Source: CAD feature listing. Evaluate the final solid. Frame: model axes, mm. Face numbers are marked on the shaded views. Give positions to 0.01 mm unless a question says otherwise; leave off trailing zeros. Loops run counter-clockwise (first coordinate to the right, second up) from the corner with the lowest first, then second, coordinate; pieces in that order, holes last. Notation, with made-up numbers: (-32.5, 27.25) -> (9.5, 27.25) arc R24 cw to (9.5, 40.25) -> close; hole circle Ø3 at (49, 20.25). An arc over 180 degrees is marked (long way). Return JSON: item names as keys, results as strings. Group by question number.
(1) Pin query (flat end, axial travel): pin 1 (2 mm diameter, centred on x = -2, z = -3, fed in from -Y); pin 2 (8 mm diameter, centred on x = -12, z = 10, fed in from +Y); pin 3 (1.5 mm diameter, centred on x = 9.5, z = 0.5, fed in from +Y); pin 4 (1.5 mm diameter, centred on y = -4, z = -7, fed in from -X). Return the tip coordinate at first contact, or that it passes through.
(2) Ray query, line 1 (X direction, y = -21, z = -13.25); line 2 (Y direction, x = -4, z = 13.5); line 3 (Z direction, x = -0.5, y = -0.75). Return the intervals inside material, ascending. Write a range as from..to.
(3) Cut plane A-A on y = -26. Return loops of the section in (x, z).
(4) Cut plane B-B on x = 11.5. Return loops of the section in (y, z).
(5) Draft query along X for the marked faces 1, 2 and 3. Return one class per face: released by +X, released by -X, zero draft, split by the parting line, or undercut.
```python
from build123d import *

# Parameters (mm, degrees)
F0_W      = 30
F0_H      = 30
F1_DEPTH  = 30
F2_W      = 25
F2_H      = 25
F2_W_2    = 17
F2_H_2    = 17
F2_W_3    = 11
F2_H_3    = 11
F2_W_4    = 3
F2_H_4    = 3
F3_DEPTH  = 2
F4_W      = 25
F4_H      = 25
F4_W_2    = 17
F4_H_2    = 17
F4_W_3    = 11
F4_H_3    = 11
F4_W_4    = 3
F4_H_4    = 3
F5_DEPTH  = 2
F6_W      = 25
F6_H      = 25
F6_W_2    = 17
F6_H_2    = 17
F6_W_3    = 11
F6_H_3    = 11
F6_W_4    = 3
F6_H_4    = 3
F7_DEPTH  = 2
F8_W      = 25
F8_H      = 25
F8_W_2    = 17
F8_H_2    = 17
F8_W_3    = 11
F8_H_3    = 11
F8_W_4    = 3
F8_H_4    = 3
F9_DEPTH  = 2
F10_W     = 25
F10_H     = 25
F10_W_2   = 17
F10_H_2   = 17
F10_W_3   = 11
F10_H_3   = 11
F10_W_4   = 3
F10_H_4   = 3
F11_DEPTH = 2
F12_W     = 25
F12_H     = 25
F12_W_2   = 17
F12_H_2   = 17
F12_W_3   = 11
F12_H_3   = 11
F12_W_4   = 3
F12_H_4   = 3
F13_DEPTH = 2


# Not quite as in the source:
# - a feature names something its author has since deleted; it is built from what else it names


with BuildPart() as f1:
    # F0 (on Front) → F1 (new body)
    with BuildSketch(Plane.XZ):
        Rectangle(F0_W, F0_H)
    extrude(amount=F1_DEPTH)

    # F2 (on face) → F3 (cut)
    with BuildSketch(Plane.XY.offset(15)):
        with Locations((0, -15)):
            Rectangle(F2_W, F2_H)
        with Locations((0, -15)):
            Rectangle(F2_W_2, F2_H_2, mode=Mode.SUBTRACT)
        with Locations((0, -15)):
            Rectangle(F2_W_3, F2_H_3)
        with Locations((0, -15)):
            Rectangle(F2_W_4, F2_H_4, mode=Mode.SUBTRACT)
    extrude(amount=-F3_DEPTH, mode=Mode.SUBTRACT)

    # F4 (on face) → F5 (cut)
    with BuildSketch(Plane(origin=(-15, 0, 0), x_dir=(0, -1, 0), z_dir=(-1, 0, 0))):
        with Locations((15, 0)):
            Rectangle(F4_W, F4_H)
        with Locations((15, 0)):
            Rectangle(F4_W_2, F4_H_2, mode=Mode.SUBTRACT)
        with Locations((15, 0)):
            Rectangle(F4_W_3, F4_H_3)
        with Locations((15, 0)):
            Rectangle(F4_W_4, F4_H_4, mode=Mode.SUBTRACT)
    extrude(amount=-F5_DEPTH, mode=Mode.SUBTRACT)

    # F6 (on face) → F7 (cut)
    with BuildSketch(Plane(origin=(0, 0, -15), x_dir=(1, 0, 0), z_dir=(0, 0, -1))):
        with Locations((0, 15)):
            Rectangle(F6_W, F6_H)
        with Locations((0, 15)):
            Rectangle(F6_W_2, F6_H_2, mode=Mode.SUBTRACT)
        with Locations((0, 15)):
            Rectangle(F6_W_3, F6_H_3)
        with Locations((0, 15)):
            Rectangle(F6_W_4, F6_H_4, mode=Mode.SUBTRACT)
    extrude(amount=-F7_DEPTH, mode=Mode.SUBTRACT)

    # F8 (on face) → F9 (cut)
    with BuildSketch(Plane.XZ.offset(30)):
        Rectangle(F8_W, F8_H)
        Rectangle(F8_W_2, F8_H_2, mode=Mode.SUBTRACT)
        Rectangle(F8_W_3, F8_H_3)
        Rectangle(F8_W_4, F8_H_4, mode=Mode.SUBTRACT)
    extrude(amount=-F9_DEPTH, mode=Mode.SUBTRACT)

    # F10 (on face) → F11 (cut)
    with BuildSketch(Plane(origin=(0, 0, 0), x_dir=(-1, 0, 0), z_dir=(0, 1, 0))):
        Rectangle(F10_W, F10_H)
        Rectangle(F10_W_2, F10_H_2, mode=Mode.SUBTRACT)
        Rectangle(F10_W_3, F10_H_3)
        Rectangle(F10_W_4, F10_H_4, mode=Mode.SUBTRACT)
    extrude(amount=-F11_DEPTH, mode=Mode.SUBTRACT)

    # F12 (on face) → F13 (cut)
    with BuildSketch(Plane.YZ.offset(15)):
        with Locations((-15, 0)):
            Rectangle(F12_W, F12_H)
        with Locations((-15, 0)):
            Rectangle(F12_W_2, F12_H_2, mode=Mode.SUBTRACT)
        with Locations((-15, 0)):
            Rectangle(F12_W_3, F12_H_3)
        with Locations((-15, 0)):
            Rectangle(F12_W_4, F12_H_4, mode=Mode.SUBTRACT)
    extrude(amount=-F13_DEPTH, mode=Mode.SUBTRACT)


solid = f1.part
```
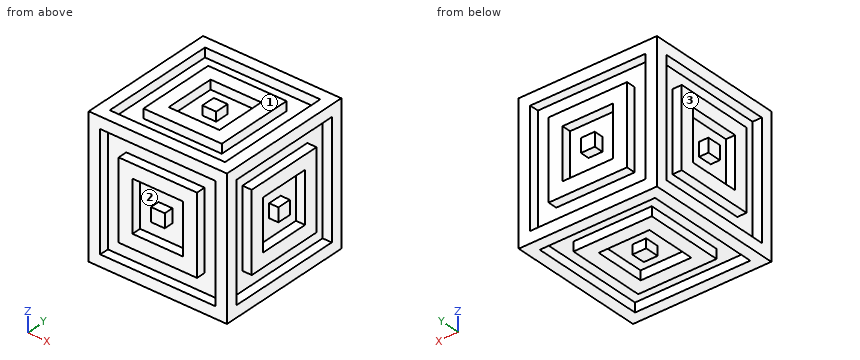
Answers:
{
 "1": {"pin 1": "y = -28", "pin 2": "y = 0", "pin 3": "y = -2", "pin 4": "x = -13"},
 "2": {"line 1": "-15..-12.5, -8.5..8.5, 12.5..15", "line 2": "-30..-27.5, -23.5..-20.5, -9.5..-6.5, -2.5..0", "line 3": "-15..-12.5, -8.5..-5.5, -1.5..1.5, 5.5..8.5, 12.5..15"},
 "3": {"outline": "(-15, -15) -> (-12.5, -15) -> (-12.5, -13) -> (12.5, -13) -> (12.5, -15) -> (15, -15) -> (15, -12.5) -> (13, -12.5) -> (13, 12.5) -> (15, 12.5) -> (15, 15) -> (12.5, 15) -> (12.5, 13) -> (-12.5, 13) -> (-12.5, 15) -> (-15, 15) -> (-15, 12.5) -> (-13, 12.5) -> (-13, -12.5) -> (-15, -12.5) -> close"},
 "4": {"outline": "(-30, -15) -> (-27.5, -15) -> (-27.5, -13) -> (-2.5, -13) -> (-2.5, -15) -> (0, -15) -> (0, -12.5) -> (-2, -12.5) -> (-2, 12.5) -> (0, 12.5) -> (0, 15) -> (-2.5, 15) -> (-2.5, 13) -> (-27.5, 13) -> (-27.5, 15) -> (-30, 15) -> (-30, 12.5) -> (-28, 12.5) -> (-28, -12.5) -> (-30, -12.5) -> close"},
 "5": {"face 1": "zero draft", "face 2": "undercut", "face 3": "released by -X"}
}
